Read the model definition and answer for the solid it produces. Units are mm, in the model's axes. Face numbers are marked on the shaded views. A direction names the side the tool comes from. Coordinates: 2 decimals unless noted, no trailing zeros. Order: outer loops, then holes, each group sorted by start corner. A loop starts at its lowest first (then second) coordinate and runs counter-clockwise, first axis right, second up.
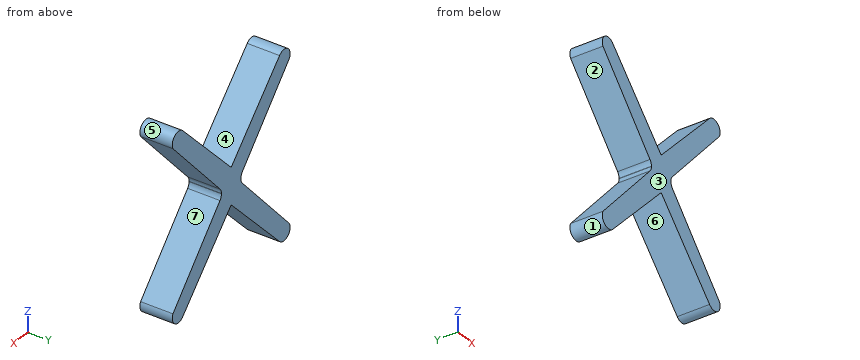
```python
from build123d import *

# Parameters (mm, degrees)
F1_DEPTH = 25.4


with BuildPart() as f1:
    # F0 (on Front) → F1 (new body)
    with BuildSketch(Plane.XZ):
        with BuildLine():
            Line((-54.477422, -71.236187), (0, -14.34601))
            Line((0, -14.34601), (54.477422, -71.236187))
            ThreePointArc((54.477422, -71.236187), (63.483736, -72.054395), (65.532006, -63.246004))
            Line((65.532006, -63.246004), (12.601703, -4.401703))
            ThreePointArc((12.601703, -4.401703), (11.393994, -2.42924), (10.9728, -0.155088))
            Line((10.9728, -0.155088), (10.9728, 0.155088))
            ThreePointArc((10.9728, 0.155088), (11.393994, 2.42924), (12.601703, 4.401703))
            Line((12.601703, 4.401703), (65.532006, 63.246004))
            ThreePointArc((65.532006, 63.246004), (63.483736, 72.054395), (54.477422, 71.236187))
            Line((54.477422, 71.236187), (0, 14.34601))
            Line((0, 14.34601), (-54.477422, 71.236187))
            ThreePointArc((-54.477422, 71.236187), (-63.483736, 72.054395), (-65.532006, 63.246004))
            Line((-65.532006, 63.246004), (-12.601703, 4.401703))
            ThreePointArc((-12.601703, 4.401703), (-11.393994, 2.42924), (-10.9728, 0.155088))
            Line((-10.9728, 0.155088), (-10.9728, -0.155088))
            ThreePointArc((-10.9728, -0.155088), (-11.393994, -2.42924), (-12.601703, -4.401703))
            Line((-12.601703, -4.401703), (-65.532006, -63.246004))
            ThreePointArc((-65.532006, -63.246004), (-63.483736, -72.054395), (-54.477422, -71.236187))
        make_face()
    extrude(amount=F1_DEPTH)


solid = f1.part
```
1) Straight lines are drawn through the part: line 1 (X direction, y = -12.5, z = 17); line 2 (X direction, y = -11.5, z = -60); line 3 (Z direction, x = -46, y = -8.75). For each, find the intervals that lie inside material, in ascending order.
A:
line 1: x = -23.93 to -2.54, 2.54 to 23.93
line 2: x = -62.61 to -43.72, 43.72 to 62.61
line 3: z = -62.38 to -41.53, 41.53 to 62.38
2) A cutting plane is placed at A-A, the plane z = -48.5. Determine the outline of the cut face in (x, y).
A:
outline: (-52.27, -25.4) - (-32.71, -25.4) - (-32.71, 0) - (-52.27, 0) - close; (32.71, -25.4) - (52.27, -25.4) - (52.27, 0) - (32.71, 0) - close
3) A cutting plane is placed at B-B, the plane x = -23. Determine the outline of the cut face in (y, z), and give its area (3 significant figures).
A:
outline: (-25.4, -38.36) - (0, -38.36) - (0, -15.96) - (-25.4, -15.96) - close; (-25.4, 15.96) - (0, 15.96) - (0, 38.36) - (-25.4, 38.36) - close
area: 1,140 mm2
4) Flat-ended cylindrical pins translate along their axes: pin 1 Ø10 at (y, z) = (-8, -58) entering from +X; pin 2 Ø1 at (y, z) = (-21, -21.5) entering from -X; pin 3 Ø4 at (x, y) = (-15.5, -22.5) entering from -Z; pin 4 Ø12 at (x, z) = (24.5, 43.5) entering from -Y. Find the tip coordinate at first contact, or state that the pin passes through.
A:
pin 1: stops at x = 65.31
pin 2: stops at x = -28.43
pin 3: stops at z = -32.62
pin 4: stops at y = -25.4
5) A cutting plane is placed at D-D, the plane z = -7. Determine the outline of the cut face in (x, y), and give its area (3 significant figures).
A:
outline: (-14.94, -25.4) - (14.94, -25.4) - (14.94, 0) - (-14.94, 0) - close
area: 759 mm2
6) Which of the six approach directions +Z, -Z, +X, -X, +Y, -Y give full straight-line access (tool end or side, diameter ignored) to the marked faces 4, 5, 6 and 7?
A:
face 4: +Z, +Y, -Y
face 5: +Y, -Y
face 6: -Z, +Y, -Y
face 7: +X, +Y, -Y
7) A cutting plane is placed at C-C, the plane y = -5.75. Determine the outline of the cut face in (x, z).
A:
outline: (-65.53, -63.25) arc R6.89 ccw to (-54.48, -71.24) - (0, -14.35) - (54.48, -71.24) arc R6.89 ccw to (65.53, -63.25) - (12.6, -4.4) arc R6.35 cw to (10.97, -0.16) - (10.97, 0.16) arc R6.35 cw to (12.6, 4.4) - (65.53, 63.25) arc R6.89 ccw to (54.48, 71.24) - (0, 14.35) - (-54.48, 71.24) arc R6.89 ccw to (-65.53, 63.25) - (-12.6, 4.4) arc R6.35 cw to (-10.97, 0.16) - (-10.97, -0.16) arc R6.35 cw to (-12.6, -4.4) - close
8) Determine the mould class of the marked faces 1, 2 and 3 for opening direction X: pulls with the +X half, pulls with the -X half, needs draft (parallel to the pull), parting line crosses it, or undercut.
A:
face 1: undercut
face 2: pulls with the -X half
face 3: needs draft
